Model file for the job. Use its own axes, mm. Round coordinates to 2 decimals unless told otherwise and drop trailing zeros. Order: outer loops, then holes, each group sorted by start corner. A loop starts at its lowest first (then second) coordinate and runs counter-clockwise, first axis right, second up. Notation, with made-up numbers: (-39.5, 31.5) - (1.5, 31.5) arc R24 ccw to (1.5, 64.5) - close; hole circle Ø9 at (35.25, 11.5). An arc over 180 degrees is marked (long way). Put each result on its own line as item: value. Start each with the question number.
Item 1: Mould opens along Z. For faces 1 (the face through (7.6, 4.03, 10.27)), 2 (the face through (7, 5, 0)), 3 (the face through (0, 5, 16)), 4 (the face through (4.805, 5.07, 26.513)) say: pulls with the +Z half, pulls with the -Z half, needs draft (parallel to the pull), parting line crosses it, or undercut.
Item 2: Pin check, flat tip, straight feed: pin 1 Ø1.9 at (y, z) = (5, 24) entering from -X (3 decimals). Stop position of the tip, or through.
Item 3: Saw through at B-B on z = 28. List the corners of the cut face in (x, y).
Item 4: Saw through at A-A on x = 5. List the corners of the cut face in (y, z), plus the area to 3 significant figures.
Item 5: Saw through at C-C on y = 4. List the corners of the cut face in (x, z).
Item 6: Probe probe 1 along Z at (x, y) = (5, 7.25); probe 2 along Y at (x, z) = (9.75, 9); probe 3 along X at (y, z) = (6, 5). List the from-to ranges inside material, lowest first.
Item 7: Saw through at D-D on x = 2.5. List the corners of the cut face in (y, z), plus the area to 3 significant figures.
Autodesk Inventor part; units mm, degrees
ref_plane "YZ Plane" through (0, 0, 0) normal (1, 0, 0) x (0, 1, 0)
ref_plane "XZ Plane" through (0, 0, 0) normal (0, 1, 0) x (-1, 0, 0)
ref_plane "XY Plane" through (0, 0, 0) normal (0, 0, 1) x (1, 0, 0)
sketch "Sketch1" plane through (0, 0, 0) normal (0, 0, 1) x (1, 0, 0)
  line L0 (0, 0) -> (15, 0)
  line L1 (15, 0) -> (15, 10)
  line L2 (15, 10) -> (0, 10)
  line L3 (0, 10) -> (0, 0)
  line L4 (1, 9) -> (14, 9)
  line L5 (14, 9) -> (14, 1)
  line L6 (14, 1) -> (1, 1)
  line L7 (1, 1) -> (1, 9)
  dimension "d0" = 15
  dimension "d1" = 10
  dimension "d2" = 13
  dimension "d3" = 8
  dimension "d4" = 1
  dimension "d5" = 1
extrude "Extrusion1" add sketch "Sketch1" along normal blind 33 contours L3 L2 L1 L0 | L4 L5 L6 L7
sketch "Sketch2" plane through (0, 10, 0) normal (0, 1, 0) x (1, 0, 0)
  line L0 (15, 0) -> (0, 0)
  line L1 (0, 0) -> (0, -33)
  line L2 (15, -33) -> (0, -33)
  line L3 (15, 0) -> (15, -33)
  circle A0 centre (5, -5) radius 1.5
  circle A1 centre (5, -28) radius 1.5
  dimension "d8" = 3
  dimension "d9" = 3
  dimension "d10" = 5
  dimension "d11" = 5
  dimension "d12" = 5
  dimension "d13" = 5
extrude "Extrusion2" cut sketch "Sketch2" against normal up to surface (10 mm away) contours A0 | A1
sketch "Sketch3" plane through (15, 0, 0) normal (1, 0, 0) x (0, 0, -1)
  line L0 (0, 0) -> (0, 10)
  line L1 (0, 10) -> (-33, 10)
  line L2 (-33, 0) -> (-33, 10)
  line L3 (0, 0) -> (-33, 0)
  circle A0 centre (-9, 5) radius 1.6
  circle A1 centre (-24, 5) radius 1.6
  dimension "d16" = 3.2
  dimension "d17" = 5
  dimension "d18" = 9
  dimension "d21" = 3.2
  dimension "d22" = 5
  dimension "d23" = 9
extrude "Extrusion3" cut sketch "Sketch3" against normal up to surface (15 mm away) contours A0 | A1
properties part number "profile2_3D" material "Aluminum 6061, Welded"
Results found:
1. face 1: undercut
1. face 2: pulls with the -Z half
1. face 3: needs draft
1. face 4: undercut
2. pin 1: passes through
3. outline: (0, 0) - (3.5, 0) - (3.5, 10) - (0, 10) - close; (6.5, 0) - (15, 0) - (15, 10) - (6.5, 10) - close
4. outline: (0, 0) - (10, 0) - (10, 3.5) - (0, 3.5) - close; (0, 6.5) - (10, 6.5) - (10, 26.5) - (0, 26.5) - close; (0, 29.5) - (10, 29.5) - (10, 33) - (0, 33) - close; hole circle Ø3.2 at (5, 9); hole circle Ø3.2 at (5, 24)
4. area: 254 mm²
5. outline: (0, 0) - (15, 0) - (15, 7.75) - (0, 7.75) - close; (0, 10.25) - (15, 10.25) - (15, 22.75) - (0, 22.75) - close; (0, 25.25) - (15, 25.25) - (15, 33) - (0, 33) - close; hole circle Ø3 at (5, 5); hole circle Ø3 at (5, 28)
6. probe 1: z = 0 to 3.5, 6.5 to 26.5, 29.5 to 33
6. probe 2: y = 0 to 3.4, 6.6 to 10
6. probe 3: x = 0 to 3.5, 6.5 to 15
7. outline: (0, 0) - (10, 0) - (10, 33) - (0, 33) - close; hole circle Ø3.2 at (5, 9); hole circle Ø3.2 at (5, 24)
7. area: 314 mm²
